```python
from build123d import *

# Parameters (mm, degrees)
SKETCH_1_R      = 18.4
SKETCH_1_R_2    = 1.5
EXTRUDE_1_DEPTH = 6.5


with BuildPart() as part:
    # Sketch 1 → Extrude 1 (new body)
    # profile 1 of 3: a face of its own
    with BuildSketch(Plane.XY):
        with Locations((0.819984335, -1.863162877)):
            Circle(SKETCH_1_R)
        with Locations(Location((14.243378094, -9.613162877, 0), (0, 0, 180))):
            Circle(SKETCH_1_R_2, mode=Mode.SUBTRACT)
        with Locations(Location((14.243378094, 5.886837123, 0), (0, 0, 180))):
            Circle(SKETCH_1_R_2, mode=Mode.SUBTRACT)
        with Locations(Location((0.819984335, 13.636837123, 0), (0, 0, 180))):
            Circle(SKETCH_1_R_2, mode=Mode.SUBTRACT)
        with Locations(Location((-12.603409424, 5.886837123, 0), (0, 0, 180))):
            Circle(SKETCH_1_R_2, mode=Mode.SUBTRACT)
        with Locations(Location((-12.603409424, -9.613162877, 0), (0, 0, 180))):
            Circle(SKETCH_1_R_2, mode=Mode.SUBTRACT)
        with Locations(Location((0.819984335, -17.363162877, 0), (0, 0, 180))):
            Circle(SKETCH_1_R_2, mode=Mode.SUBTRACT)
        with BuildLine():
            ThreePointArc((-6.180015665, 4.386837123), (-12.430015665, -1.863162877), (-6.180015665, -8.113162877))
            Line((-6.180015665, -8.113162877), (7.819984335, -8.113162877))
            ThreePointArc((7.819984335, -8.113162877), (14.069984335, -1.863162877), (7.819984335, 4.386837123))
            Line((7.819984335, 4.386837123), (-6.180015665, 4.386837123))
        make_face(mode=Mode.SUBTRACT)
    # profile 2 of 3: a face of its own
    with BuildSketch(Plane.XY):
        with BuildLine():
            Line((-17.580015665, 16.536837123), (-17.580015665, -1.863163013))
            ThreePointArc((-17.580015665, -1.863163013), (-12.190780487, 11.147601849), (0.819984335, 16.536837123))
            Line((0.819984335, 16.536837123), (-17.580015665, 16.536837123))
        make_face()
    # profile 3 of 3: a face of its own
    with BuildSketch(Plane.XY):
        with BuildLine():
            Line((-17.580015665, -20.263162877), (0.819984335, -20.263162877))
            ThreePointArc((0.819984335, -20.263162877), (-12.190780391, -14.873927699), (-17.580015665, -1.863163013))
            Line((-17.580015665, -1.863163013), (-17.580015665, -20.263162877))
        make_face()
    extrude(amount=EXTRUDE_1_DEPTH)


solid = part.part
```
Can you work these out from the model? Positions are in its coordinate system, mm. A direction names the side the tool comes from. Coordinates: 2 decimals unless noted, no trailing zeros. Loops run counter-clockwise (first coordinate to the right, second up) from the corner with the lowest first, then second, coordinate; pieces in that order, holes last. Notation, with made-up numbers: (86, 35.5) -> (136, 35.5) arc R26 cw to (136, 59.5) -> close; hole circle Ø3 at (58, 72.25). An arc over 180 degrees is marked (long way). Put each result on its own line as item: value. Start each with the question number.
Q1. Thinking about a two-plate mould opening in Y: for faces 1 (the face through (-8, 16.537, 3)), 2 (the face through (-9, -20.263, 3)), 3 (the face through (-12.43, -1.73, 3.2)), which applies, pulls with the +Y half, pulls with the -Y half, needs draft (parallel to the pull), parting line crosses it, or undercut?
Q2. For faces 4 (the face through (14.07, -2, 3.2)), 5 (the face through (1, -10, 0)), which set-ups out of +Z, -Z, +X, -X, +Y, -Y let a thin tool reach every point of the face, with its end or its side?
Q3. I want a section at C-C (y = -9). Write out the boundary of the cut face in (x, z), plus the area to 3 significant figures.
Q4. If I drill on line 1 (Y direction, x = -4.5, z = 0.75); line 2 (Y direction, x = -13.5, z = 4.5); line 3 (X direction, y = -9, z = 3.5), over which ranges is the centre line in solid material (lowest first)? Write a range as [from, to].
Q5. I want a section at A-A (x = -2.5). Write out the boundary of the cut face in (y, z).
Q6. I'm going to push a flat-ended pin straight in: P1, Ø3, axis at x = 3, z = 3, coming from the -Y side. Where does the tip first touch, or does it pass through?
Q7. I want a section at B-B (y = 1). Write out the boundary of the cut face in (x, z), plus the area to 3 significant figures.
Q8. I want a section at D-D (x = 13.5). Write out the boundary of the cut face in (y, z).
Taken from the geometry:
1. face 1: pulls with the +Y half
1. face 2: pulls with the -Y half
1. face 3: undercut
2. face 4: +Z, -Z
2. face 5: -Z, +X, -X, +Y, -Y
3. outline: (-17.58, 0) -> (-13.97, 0) -> (-13.97, 6.5) -> (-17.58, 6.5) -> close; (-11.23, 0) -> (12.87, 0) -> (12.87, 6.5) -> (-11.23, 6.5) -> close; (15.61, 0) -> (17.78, 0) -> (17.78, 6.5) -> (15.61, 6.5) -> close
3. area: 194 mm2
4. line 1: y = [-20.26, -8.11], [4.39, 16.54]
4. line 2: y = [-20.26, -10.82], [-8.41, 4.68], [7.09, 16.54]
4. line 3: x = [-17.58, -13.97], [-11.23, 12.87], [15.61, 17.78]
5. outline: (-20.26, 0) -> (-8.11, 0) -> (-8.11, 6.5) -> (-20.26, 6.5) -> close; (4.39, 0) -> (16.54, 0) -> (16.54, 6.5) -> (4.39, 6.5) -> close
6. P1: stops at y = -20.25
7. outline: (-17.58, 0) -> (-11.74, 0) -> (-11.74, 6.5) -> (-17.58, 6.5) -> close; (13.38, 0) -> (19, 0) -> (19, 6.5) -> (13.38, 6.5) -> close
7. area: 74.5 mm2
8. outline: (-15.2, 0) -> (-10.92, 0) -> (-10.92, 6.5) -> (-15.2, 6.5) -> close; (-8.31, 0) -> (-4.47, 0) -> (-4.47, 6.5) -> (-8.31, 6.5) -> close; (0.74, 0) -> (4.58, 0) -> (4.58, 6.5) -> (0.74, 6.5) -> close; (7.19, 0) -> (11.47, 0) -> (11.47, 6.5) -> (7.19, 6.5) -> close
